For this review, use the dimensioned drawing (mm, ordinates from the lowest corner) and the shaded views. Coordinates: 2 decimals unless noted, no trailing zeros. Loops run counter-clockwise (first coordinate to the right, second up) from the corner with the lowest first, then second, coordinate; pieces in that order, holes last.
1. Take a section at B-B, the plane y = 31. State the section outline as (x, z) points, then the cut area to 3 significant figures.
2. Clearance check with flat-ended pins moving along their axes: P1, Ø1.9, axis at x = 5.5, z = 2, coming from the -Y side; P2, Ø1.9, axis at y = 11, z = 2, coming from the +X side; P3, Ø3, axis at x = 93, z = 4.5, coming from the -Y side; P4, Ø8, axis at x = 85, y = 115, coming from the -Z side. State where each tip first meets the part, or that it passes through.
3. Take a section at C-C, the plane x = 23. State the section outline as (y, z) points, then the cut area to 3 significant figures.
4. To check wall thickness, follow probe 1 along Y at (x, z) = (90, 1); probe 2 along X at (y, z) = (86, 5.5); probe 3 along Y at (x, z) = (44, 2.25). State the ranges of each line that lie inside material, in increasing order.
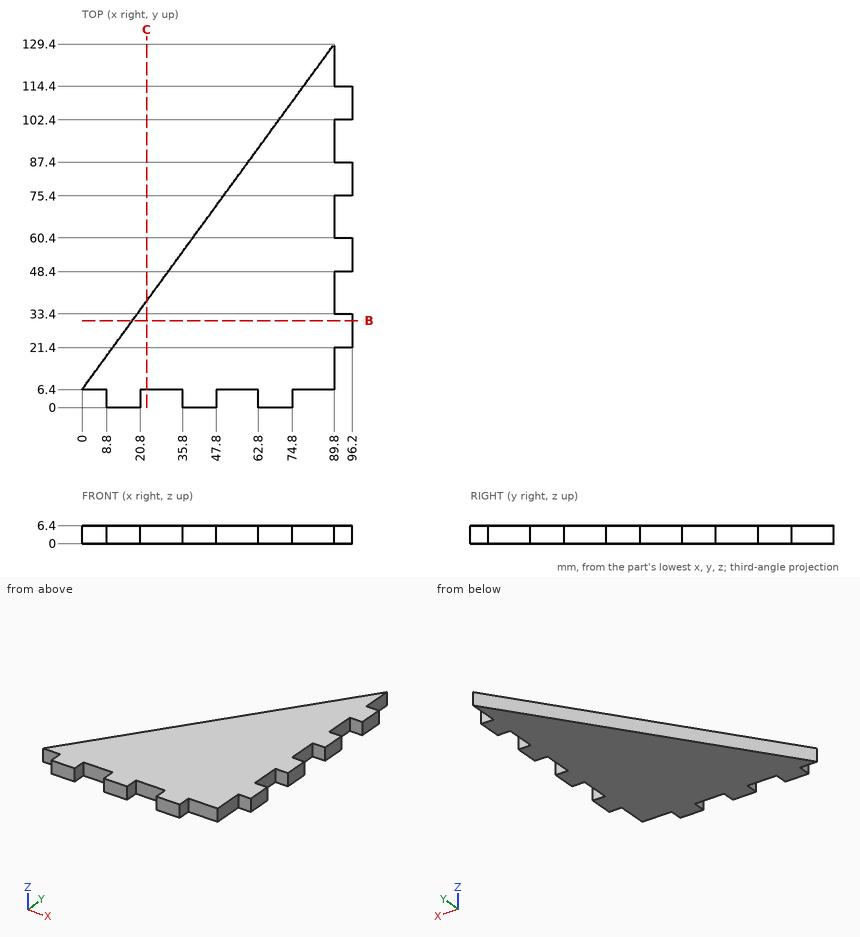
Results list:
1. outline: (17.96, 0) - (96.2, 0) - (96.2, 6.4) - (17.96, 6.4) - close
1. area: 501 mm2
2. P1: stops at y = 6.4
2. P2: stops at x = 89.8
2. P3: stops at y = 21.4
2. P4: stops at z = 0
3. outline: (6.4, 0) - (37.9, 0) - (37.9, 6.4) - (6.4, 6.4) - close
3. area: 202 mm2
4. probe 1: y = 21.4 to 33.4, 48.4 to 60.4, 75.4 to 87.4, 102.4 to 114.4
4. probe 2: x = 58.11 to 96.2
4. probe 3: y = 0 to 66.67
